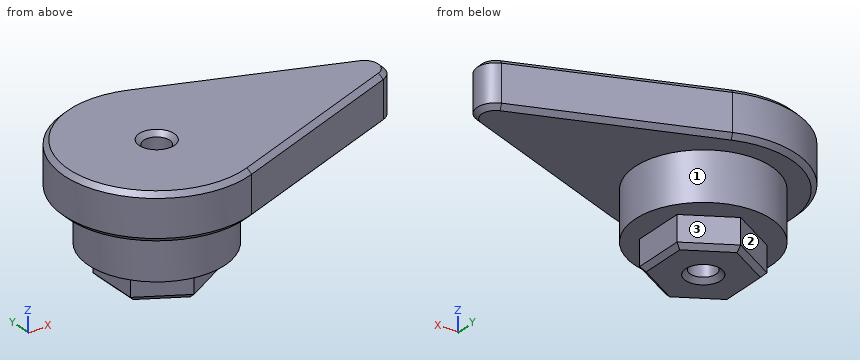
```python
from build123d import *

# Parameters (mm, degrees)
PAD003_DEPTH    = 6.5
SKETCH007_R     = 14.75
PAD004_DEPTH    = 10.5
PAD005_DEPTH    = 10
SKETCH009_R     = 2.8
POCKET002_DEPTH = 27.001
CHAMFER_SIZE    = 1


with BuildPart() as part:
    # Sketch006 → Pad003 (new body)
    with BuildSketch(Plane.XY):
        Polygon((0, -11.25833), (9.75, -5.629165), (9.75, 5.629165), (0, 11.25833), (-9.75, 5.629165), (-9.75, -5.629165), align=None)
    extrude(amount=PAD003_DEPTH)

    # Sketch007 (on Face8 of Pad003) → Pad004 (join)
    with BuildSketch(Plane.XY.offset(6.5)):
        Circle(SKETCH007_R)
    extrude(amount=PAD004_DEPTH)

    # Sketch008 (on Face3 of Pad004) → Pad005 (join)
    with BuildSketch(Plane.XY.offset(17)):
        with BuildLine():
            ThreePointArc((7.111111, 18.693103), (-20, 0), (7.111111, -18.693103))
            Line((46.422222, -3.738621), (7.111111, -18.693103))
            ThreePointArc((46.422222, -3.738621), (49, 0), (46.422222, 3.738621))
            Line((46.422222, 3.738621), (7.111111, 18.693103))
        make_face()
    extrude(amount=PAD005_DEPTH)

    # Sketch009 (on Face5 of Pad005) → Pocket002 (cut, through all)
    with BuildSketch(Plane.XY.offset(27)):
        Circle(SKETCH009_R)
    extrude(amount=-POCKET002_DEPTH, mode=Mode.SUBTRACT)

    # Chamfer
    chamfer_edges = [part.edges().sort_by_distance(p)[0] for p in [
        (49, 0, 27),
        (26.766667, -11.215862, 27),
        (26.766667, 11.215862, 27),
        (-20, 0, 27),
        (-2.8, 0, 27),
        (26.766667, -11.215862, 17),
        (4.875, -8.443748, 0),
        (-4.875, -8.443748, 0),
        (9.75, 0, 0),
        (-9.75, 0, 0),
        (4.875, 8.443748, 0),
        (-4.875, 8.443748, 0),
        (-2.8, 0, 0),
    ]]
    chamfer(chamfer_edges, length=CHAMFER_SIZE)


with BuildPart() as part_1:
    # Body002 placement: moved
    add(part.part.moved(Location((0, 12, 0))))


solid = part_1.part
```
The model under review builds one solid part; all positions refer to its coordinate system, in mm. Face numbers are marked on the shaded views. A direction names the side the tool comes from. Round coordinates to 2 decimals unless told otherwise and drop trailing zeros. Order: outer loops, then holes, each group sorted by start corner. A loop starts at its lowest first (then second) coordinate and runs counter-clockwise, first axis right, second up.
(1) Take a section at D-D, the plane z = 13.5. State the section outline as (x, y) points.
Working result:
outline: circle Ø29.5 at (0, 12); hole circle Ø5.6 at (0, 12)
(2) Take a section at B-B, the plane z = 24.75. State the section outline as (x, y) points.
Working result:
outline: (7.11, -6.69) - (46.42, 8.26) arc R4 ccw to (46.42, 15.74) - (7.11, 30.69) arc R20 ccw (long way) to start; hole circle Ø5.6 at (0, 12)
(3) For P1, Ø4, axis at y = 15.5, z = 21.5, coming from the +X side; P2, Ø12, axis at x = -7, z = 20.5, coming from the +Y side (3 decimals); P3, Ø6, axis at y = 17, z = 13.5, coming from the +X side; P4, Ø5, axis at x = 0, y = 12, coming from the -Z side, all flat-tipped, find the tip position at first contact; note any pin that passes through.
Working result:
P1: stops at x = 48.71
P2: stops at y = 31.975
P3: stops at x = 14.61
P4: passes through
(4) Take a section at C-C, the plane x = 19. State the section outline as (y, z) points, plus the area to 3 significant figures.
Working result:
outline: (-2.17, 18) - (-1.1, 17) - (25.1, 17) - (26.17, 18) - (26.17, 26) - (25.1, 27) - (-1.1, 27) - (-2.17, 26) - close
area: 281 mm2
(5) Wall thickness on L1, parallel to Y at x = 0, z = 8.5; L2, parallel to Z at x = 17, y = 23.5; L3, parallel to Z at x = 9, y = 5: over which ranges is each line inside the solid? List them lowest first.
Working result:
L1: y = -2.75 to 9.2, 14.8 to 26.75
L2: z = 17 to 27
L3: z = 6.5 to 27
(6) Tool access review of the marked faces 1, 2 and 3: name each direction out of +Z, -Z, +X, -X, +Y, -Y from which nothing blocks a thin tool from reaching the whole face with its end or side.
Working result:
face 1: -Z
face 2: -Z, -X, +Y
face 3: -Z, +X, +Y
(7) Take a section at A-A, the plane y = 12. State the section outline as (x, z) points, plus the area to 3 significant figures.
Working result:
outline: (-20, 18) - (-19, 17) - (-14.75, 17) - (-14.75, 6.5) - (-9.75, 6.5) - (-9.75, 1) - (-8.75, 0) - (-3.8, 0) - (-2.8, 1) - (-2.8, 26) - (-3.8, 27) - (-19, 27) - (-20, 26) - close; (2.8, 1) - (3.8, 0) - (8.75, 0) - (9.75, 1) - (9.75, 6.5) - (14.75, 6.5) - (14.75, 17) - (48, 17) - (49, 18) - (49, 26) - (48, 27) - (3.8, 27) - (2.8, 26) - close
area: 970 mm2
